Source: CAD feature listing. Evaluate the final solid. Frame: model axes, mm. Face numbers are marked on the shaded views. A direction names the side the tool comes from. Give positions to 0.01 mm unless a question says otherwise; leave off trailing zeros. Write each loop counter-clockwise with the first axis right and the second up, starting at its lowest first coordinate (ties: lowest second). Pieces come first, ordered by that corner, then holes.
```python
from build123d import *

# Parameters (mm, degrees)
F1_DEPTH       = 32.5
F2_W           = 40
F2_H           = 15
F3_DEPTH       = 40.001
F3_DEPTH_BACK  = 40.001
F4_R           = 4.99999
F6_D           = 5.5
F6_START       = 4.9375
F6_START_2     = 4.9723205
F6_CBORE_D     = 9.75
F6_CBORE_DEPTH = 1
F7_W           = 5
F7_H           = 12
F8_DEPTH       = 0.5358983849
F9_T4_DEPTH    = 13.5430097928
F9_T10_DEPTH   = 13.5430097928


# Not quite as in the source:
# - a fillet or chamfer that OpenCascade refuses, or shapes differently, is made with other operations: its cross-section is extruded or revolved along the edge and cut away or added
# - a fillet or chamfer is up to 0.001 mm smaller than in the source, because OpenCascade refuses the exact size


with BuildPart() as f1:
    # F0 (on Right) → F1 (new body, symmetric)
    with BuildSketch(Plane.YZ):
        Polygon((0, 10), (0, 20), (-10, 20), (-40, 5), (-40, 0), (40, 0), (40, 5), (15, 10.5358983849), (12, 10.5358983849), (10, 10), align=None)
    extrude(amount=F1_DEPTH, both=True)

    # F2 (on Front) → F3 (cut, two sides)
    with BuildSketch(Plane.XZ) as f3_sk:
        with Locations((0, 12.5)):
            Rectangle(F2_W, F2_H)
    extrude(amount=-F3_DEPTH, mode=Mode.SUBTRACT)
    extrude(f3_sk.sketch, amount=F3_DEPTH_BACK, mode=Mode.SUBTRACT)

    # F4 (radius 5 in the source; OpenCascade refuses exactly that, so slightly less here)
    f4_edges = [f1.edges().sort_by_distance(p)[0] for p in [
        (20, 0, 5),
        (-20, 0, 5),
    ]]
    fillet(f4_edges, radius=F4_R)

    # F6 (through all)
    # its depths count from where the whole tool has entered the part; down to there all is cleared
    with Locations(Plane.XY.offset(10)):
        with Locations((-26.25, 35, -F6_START_2), (26.25, 35, -F6_START_2), (-26.25, -35, -F6_START), (26.25, -35, -F6_START)):
            CounterBoreHole(F6_D / 2, F6_CBORE_D / 2, F6_CBORE_DEPTH)

    # F7 (on face) → F8 (join, through all)
    with BuildSketch(Plane.XY.offset(10)):
        with Locations((-30, 6)):
            Rectangle(F7_W, F7_H)
        with Locations((30, 6)):
            Rectangle(F7_W, F7_H)
    extrude(amount=F8_DEPTH)

    # F9: chamfer of 0.6 on 2 edges, made by hand


with BuildPart() as f9_tool2:
    # F9_s3 → F9_t4 (new body)
    with BuildSketch(Plane.XZ.offset(-13.5430097928)):
        Polygon((27.5, 9.9358983849), (28.1, 10.5358983849), (27.5, 10.5358983849), align=None)
    extrude(amount=F9_T4_DEPTH)

    split(bisect_by=Plane(origin=(0, -1.8301270189, 6.8301270189), x_dir=(1, 0, 0), z_dir=(0, -0.2588190451, 0.9659258263)), keep=Keep.TOP)

    split(bisect_by=Plane.XY.offset(10), keep=Keep.TOP)


with BuildPart() as f1_1:
    add(f1.part)

    # F9_t1: cut F9_tool2
    add(f9_tool2.part, mode=Mode.SUBTRACT)


with BuildPart() as f9_tool8:
    # F9_s9 → F9_t10 (new body)
    with BuildSketch(Plane.XZ):
        Polygon((-27.5, 9.9358983849), (-28.1, 10.5358983849), (-27.5, 10.5358983849), align=None)
    extrude(amount=-F9_T10_DEPTH)

    split(bisect_by=Plane(origin=(0, -1.8301270189, 6.8301270189), x_dir=(1, 0, 0), z_dir=(0, -0.2588190451, 0.9659258263)), keep=Keep.TOP)

    split(bisect_by=Plane.XY.offset(10), keep=Keep.TOP)


with BuildPart() as f1_2:
    add(f1_1.part)

    # F9_t7: cut F9_tool8
    add(f9_tool8.part, mode=Mode.SUBTRACT)


solid = f1_2.part
```
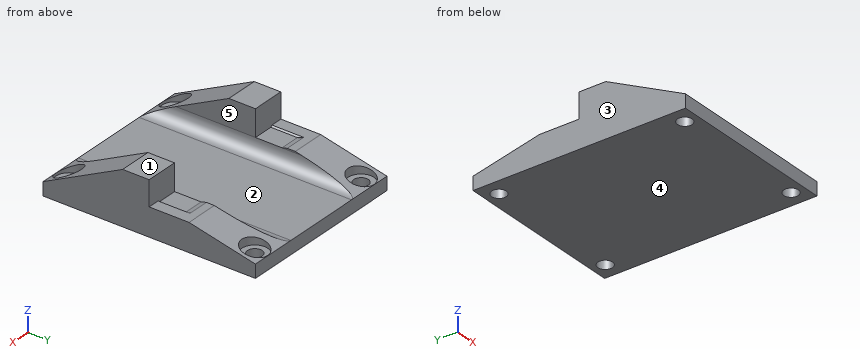
1. Cut plane C-C, the plane x = -26.25. State how many separate pieces and enclosed holes the cut face has, then the cut area to 3 significant figures.
2. Cut plane A-A, the plane z = 17.25. Return the cut outline in (x, y).
3. Access query for the marked faces 4 and 5. Directions: +Z, -Z, +X, -X, +Y, -Y. A direction counts if a zero-diameter tool reaches every point of the face in a straight line with its end or side. Return the directions, or none.
4. Line query: L1, parallel to Y at x = -26.25, z = 2.7; L2, parallel to X at y = -23.5, z = 9.75; L3, parallel to Z at x = 10.5, y = 19. Output: solid intervals per line, ascending.
5. Contact query for flat-ended pins moving along their axis: P1, Ø10.5, axis at x = 24, y = 33, coming from the +Z side; P2, Ø4, axis at x = -24, y = 5, coming from the +Z side; P3, Ø8, axis at x = 26.25, y = 35, coming from the +Z side; P4, Ø3, axis at x = -26, y = 36, coming from the +Z side. Output: stop coordinate, or through.
6. Mould query, pull axis X, two halves, no side actions, for the marked faces 1, 2 and 3. Classes: +X half, -X half, draft (parallel to the pull), parting line (faces both ways), or undercut.
7. Cut plane D-D, the plane y = 35. Return the cut outline in (x, z) (3 decimals), then the cut area to 3 significant figures.
Response values:
1. separate pieces: 3
1. enclosed holes: 0
1. area: 823 mm2
2. outline: (-32.5, -15.5) - (-20, -15.5) - (-20, 0) - (-32.5, 0) - close; (20, -15.5) - (32.5, -15.5) - (32.5, 0) - (20, 0) - close
3. face 4: -Z, +X, -X, +Y, -Y
3. face 5: +Z, +Y, -Y
4. L1: y = -40 to -37.75, -32.25 to 32.25, 37.75 to 40
4. L2: x = -32.5 to -19.99, 19.99 to 32.5
4. L3: z = 0 to 5
5. P1: stops at z = 7.71
5. P2: stops at z = 10
5. P3: stops at z = 4.03
5. P4: passes through
6. face 1: draft
6. face 2: undercut
6. face 3: -X half
7. outline: (-32.5, 0) - (-29, 0) - (-29, 4.028) - (-31.125, 4.028) - (-31.125, 6.107) - (-32.5, 6.107) - close; (-23.5, 0) - (23.5, 0) - (23.5, 4.028) - (21.375, 4.028) - (21.375, 6.107) - (18.138, 6.107) arc R5 cw to (15, 5) - (-15, 5) arc R5 cw to (-18.138, 6.107) - (-21.375, 6.107) - (-21.375, 4.028) - (-23.5, 4.028) - close; (29, 0) - (32.5, 0) - (32.5, 6.107) - (31.125, 6.107) - (31.125, 4.028) - (29, 4.028) - close
7. area: 274 mm2
